```python
from build123d import *

# Parameters (mm, degrees)
SKETCH1_R           = 77.47
SKETCH1_R_2         = 77.0128
BOSS_EXTRUDE1_DEPTH = 76.2
SKETCH2_W           = 20.32
SKETCH2_H           = 2.54
BOSS_EXTRUDE2_DEPTH = 76.2
SKETCH3_R           = 3.175
CUT_EXTRUDE3_DEPTH  = 2.54


with BuildPart() as part:
    # Sketch1 → Boss-Extrude1 (new body)
    with BuildSketch(Plane.XY):
        Circle(SKETCH1_R)
        Circle(SKETCH1_R_2, mode=Mode.SUBTRACT)
    extrude(amount=BOSS_EXTRUDE1_DEPTH)

    # Sketch2 → Boss-Extrude2 (add)
    with BuildSketch(Plane.XY.offset(76.2)):
        with Locations((87.162327652, 0)):
            Rectangle(SKETCH2_W, SKETCH2_H)
        with Locations((-87.162327652, 0)):
            Rectangle(SKETCH2_W, SKETCH2_H)
    extrude(amount=-BOSS_EXTRUDE2_DEPTH)

    # Sketch3 → Cut-Extrude3 (cut)
    with BuildSketch(Plane(origin=(0, 1.27, 0), x_dir=(1, 0, 0), z_dir=(0, 1, 0))):
        with Locations((89.995251464, -9.525)):
            Circle(SKETCH3_R)
        with Locations((89.995251464, -28.575)):
            Circle(SKETCH3_R)
        with Locations((89.995251464, -47.625)):
            Circle(SKETCH3_R)
        with Locations((89.995251464, -66.675)):
            Circle(SKETCH3_R)
        with Locations((-89.995251464, -9.525)):
            Circle(SKETCH3_R)
        with Locations((-89.995251464, -28.575)):
            Circle(SKETCH3_R)
        with Locations((-89.995251464, -47.625)):
            Circle(SKETCH3_R)
        with Locations((-89.995251464, -66.675)):
            Circle(SKETCH3_R)
    extrude(amount=-CUT_EXTRUDE3_DEPTH, mode=Mode.SUBTRACT)


solid = part.part
```
Geometry: final body of the model. Coordinates: model frame, mm. A direction names the side the tool comes from. Coordinates: 2 decimals unless noted, no trailing zeros. Loops run counter-clockwise (first coordinate to the right, second up) from the corner with the lowest first, then second, coordinate; pieces in that order, holes last. Notation, with made-up numbers: M 3.25,89.5 L 45.25,89.5 A20 ccw 45.25,117.5 Z; hole C -16,14 d8. An arc over 180 degrees is marked long. Put each result on its own line as item: value.
(1) Draft query along X for faces 1 (the face through (93.024, 0.018, 8.571)), 2 (the face through (72, -28, 76.2)), 3 (the face through (-1.69, -77.45, 37.57)). Return one class per face: pulls with the +X half, pulls with the -X half, needs draft (parallel to the pull), parting line crosses it, or undercut.
Answer sheet:
face 1: undercut
face 2: needs draft
face 3: parting line crosses it
(2) Material intervals for probe 1 along Y at (x, z) = (23, 51); probe 2 along Y at (x, z) = (-58, 31); probe 3 along X at (y, z) = (45.5, 4), sorted ascending.
Answer sheet:
probe 1: y = -73.98 to -73.5, 73.5 to 73.98
probe 2: y = -51.36 to -50.67, 50.67 to 51.36
probe 3: x = -62.7 to -62.13, 62.13 to 62.7
(3) Cut plane A-A on x = 0. Return the cut outline in (y, z).
Answer sheet:
outline: M -77.47,0 L -77.01,0 L -77.01,76.2 L -77.47,76.2 Z; M 77.01,0 L 77.47,0 L 77.47,76.2 L 77.01,76.2 Z
(4) Cut plane B-B on z = 15. Return the cut outline in (x, y), then the cut area to 3 significant figures.
Answer sheet:
outline: M -97.32,-1.27 L -77.46,-1.27 A77.47 ccw 77.46,-1.27 L 97.32,-1.27 L 97.32,1.27 L 77.46,1.27 A77.47 ccw -77.46,1.27 L -97.32,1.27 Z; hole M -77,-1.27 A77.01 ccw 77,-1.27 L 77,1.27 A77.01 ccw -77,1.27 Z
area: 323 mm^2
(5) Access query for faces 4 (the face through (1.676, 76.995, 37.567)), 5 (the face through (87, -1.27, 39)), 6 (the face through (-88, -1.27, 39)), 7 (the face through (-88, 1.27, 39)), 8 (the face through (87, 1.27, 39)). Directions: +Z, -Z, +X, -X, +Y, -Y. A direction counts if a zero-diameter tool reaches every point of the face in a straight line with its end or side. Return the directions, or none.
Answer sheet:
face 4: +Z, -Z
face 5: +Z, -Z, +X, -Y
face 6: +Z, -Z, -X, -Y
face 7: +Z, -Z, -X, +Y
face 8: +Z, -Z, +X, +Y
(6) First-contact query: pin 1 (22 mm diameter, centred on x = -92, z = 51, fed in from -Y); pin 2 (4 mm diameter, centred on x = -90, z = 66.68, fed in from -Y); pin 3 (2 mm diameter, centred on y = 35, z = 24, fed in from -X); pin 4 (22 mm diameter, centred on x = -88.5, z = 28, fed in from +Y). Flat tips, straight axial feed; report the tip coordinate or a pass-through.
Answer sheet:
pin 1: stops at y = -1.27
pin 2: passes through
pin 3: stops at x = -69.61
pin 4: stops at y = 1.27
(7) Cut plane C-C on y = 56.5. Return the cut outline in (x, z).
Answer sheet:
outline: M -53,0 L -52.33,0 L -52.33,76.2 L -53,76.2 Z; M 52.33,0 L 53,0 L 53,76.2 L 52.33,76.2 Z
